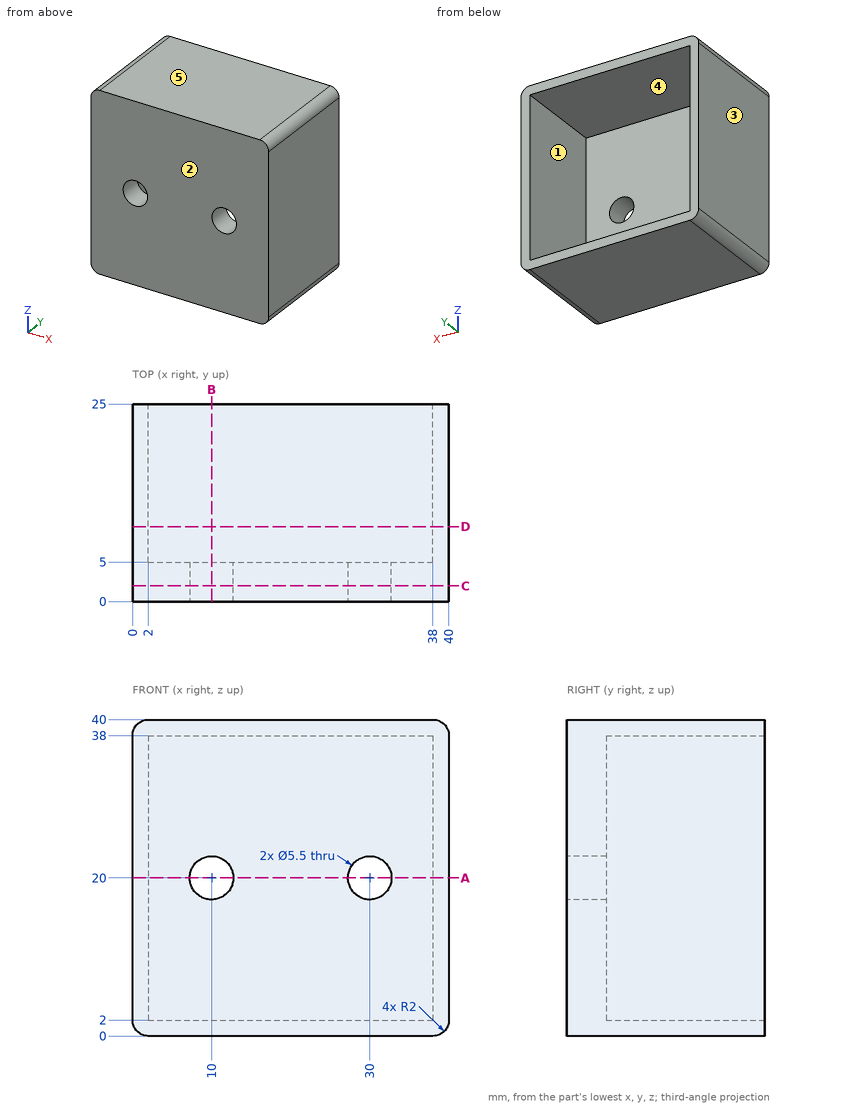
Could you check a few things on this drawing? It's one solid part, dimensions in mm from its lowest x, y, z. A direction names the side the tool comes from. Give positions to 0.01 mm unless a question says otherwise; leave off trailing zeros. Order: outer loops, then holes, each group sorted by start corner. A loop starts at its lowest first (then second) coordinate and runs counter-clockwise, first axis right, second up. Notation, with made-up numbers: M 8,49.25 L 13,49.25 A18 cw 13,77.25 Z; hole C 5.5,51 d6. An arc over 180 degrees is marked long. Use one line per item in the form item = value. Start each with the question number.
Item 1: If we section it at A-A (z = 20): Write out the boundary of the cut face in (x, y), then the cut area to 3 significant figures.
Item 2: Will this pin go through, and if not, where does the flat tip stop? pin 1 Ø6 at (x, z) = (29.5, 8.5) entering from +Y.
Item 3: If we section it at D-D (y = 9.5): Write out the boundary of the cut face in (x, z).
Item 4: We'd pull the mould along X, two halves only. Please class the marked faces 3, 4 and 5: +X half, -X half, draft (parallel to the pull), parting line (faces both ways), or undercut.
Item 5: For the marked faces 1 and 2, which set-ups out of +Z, -Z, +X, -X, +Y, -Y let a thin tool reach every point of the face, with its end or its side?
Item 6: If I drill on line 1 along X through (y, z) = (1.25, 20); line 2 along Z through (x, y) = (30, 1.7); line 3 along Z through (x, y) = (2.5, 21.25), over which ranges is the centre line in solid material (lowest first)?
Item 7: If we section it at B-B (x = 10): Write out the boundary of the cut face in (y, z), then the cut area to 4 significant figures.
Item 8: If we section it at C-C (y = 2): Write out the boundary of the cut face in (x, z).
Outcome:
q1.outline = M 0,0 L 7.25,0 L 7.25,5 L 2,5 L 2,25 L 0,25 Z; M 12.75,0 L 27.25,0 L 27.25,5 L 12.75,5 Z; M 32.75,0 L 40,0 L 40,25 L 38,25 L 38,5 L 32.75,5 Z
q1.area = 225 mm2
q2.pin_1 = 5
q3.outline = M 0,2 A2 ccw 2,0 L 38,0 A2 ccw 40,2 L 40,38 A2 ccw 38,40 L 2,40 A2 ccw 0,38 Z; hole M 2,2 L 38,2 L 38,38 L 2,38 Z
q4.face_3 = -X half
q4.face_4 = undercut
q4.face_5 = draft
q5.face_1 = +Y
q5.face_2 = +Z, -Z, +X, -X, -Y
q6.line_1 = 0 to 7.25, 12.75 to 27.25, 32.75 to 40
q6.line_2 = 0 to 17.25, 22.75 to 40
q6.line_3 = 0 to 2, 38 to 40
q7.outline = M 0,0 L 25,0 L 25,2 L 5,2 L 5,17.25 L 0,17.25 Z; M 0,22.75 L 5,22.75 L 5,38 L 25,38 L 25,40 L 0,40 Z
q7.area = 252.5 mm2
q8.outline = M 0,2 A2 ccw 2,0 L 38,0 A2 ccw 40,2 L 40,38 A2 ccw 38,40 L 2,40 A2 ccw 0,38 Z; hole C 10,20 d5.5; hole C 30,20 d5.5
